Here's how the part is built. I have some questions about the finished solid (model axes, mm). Face numbers are marked on the shaded views. A direction names the side the tool comes from. Coordinates: 2 decimals unless noted, no trailing zeros. Write each loop counter-clockwise with the first axis right and the second up, starting at its lowest first coordinate (ties: lowest second). Pieces come first, ordered by that corner, then holes. Notation, with made-up numbers: (44.5, 19) - (66.5, 19) arc R18 ccw to (66.5, 29) - close; hole circle Ø6 at (30, 5). An arc over 180 degrees is marked (long way). Answer in a Markdown table with one row per item. Add a question column.
Item 1: Imagine slicing it at D-D (z = 20). Please give me the cut outline in (x, y), plus the area to 3 significant figures.
Item 2: Imagine slicing it at B-B (y = 0). Please give me the cut outline in (x, z) (3 decimals), plus the area to 3 significant figures.
Item 3: Imagine slicing it at C-C (z = 10). Please give me the cut outline in (x, y) (3 decimals), plus the area to 3 significant figures.
Item 4: If I drill on probe 1 along X at (y, z) = (0, 10.5) (3 decimals); probe 2 along Y at (x, z) = (2, 16.5); probe 3 along Y at (x, z) = (-2, 22), over which ranges is the centre line in solid material (lowest first)? Write a range as from..to.
Item 5: Imagine slicing it at A-A (x = 0). Please give me the cut outline in (y, z) (3 decimals), plus the area to 3 significant figures.
Item 6: Which directions (+Z, -Z, +X, -X, +Y, -Y) give clear straight access to the entire face, cutting with the end or side of a thin tool? Please do the marked faces 1 and 2.
Item 7: We'd pull the mould along X, two halves only. Please class the marked faces 3, 4, 5 and 6: +X half, -X half, draft (parallel to the pull), parting line (faces both ways), or undercut.
Item 8: I'm going to push flat-ended pins straight in: pin 1 (2 mm diameter, centred on y = -17, z = 27.5, fed in from +X); pin 2 (18.5 mm diameter, centred on y = 17.5, z = 15.5, fed in from -X); pin 3 (1.5 mm diameter, centred on x = -4, y = 19.5, fed in from -Z); pin 4 (1.5 mm diameter, centred on x = 0, y = 21.5, fed in from -Z). Where does each tip first touch, or does it pass through?
from build123d import *

# Parameters (mm, degrees)
PAD_DEPTH = 2.8


with BuildPart() as pad:
    # Sketch001 → Pad (new body, symmetric)
    with BuildSketch(Plane.YZ):
        with BuildLine():
            Line((6.5, 0), (6.5, 14))
            Line((6.5, 14), (10.5, 14))
            Line((10.5, 14), (17.86865, 27.377357))
            ThreePointArc((29.028201, 19.12997), (28.160419, 29.629469), (17.86865, 27.377357))
            Line((10.5, 0), (29.028201, 19.12997))
            Line((6.5, 0), (10.5, 0))
        make_face()
        with BuildLine():
            Line((-29.028193, 19.12994), (-10.49996, 0))
            Line((-10.49996, 0), (-6.49996, 0))
            Line((-6.49996, 0), (-6.49996, 14))
            Line((-6.49996, 14), (-10.49996, 14))
            Line((-10.49996, 14), (-17.86865, 27.377335))
            ThreePointArc((-17.86865, 27.377335), (-28.160423, 29.629443), (-29.028193, 19.12994))
        make_face()
    extrude(amount=PAD_DEPTH, both=True)


with BuildPart() as obj1:
    # Sketch → Revolution (revolve)
    with BuildSketch(Plane.YZ):
        Polygon((6, 0), (5.055, 0.545596), (5.055, 13.454404), (6, 14), (8.5, 14), (10, 0), align=None)
    revolve(axis=Axis((0, 0, 0), (0, 0, 1)))

    # Fusion: union Pad
    add(pad.part)


solid = obj1.part
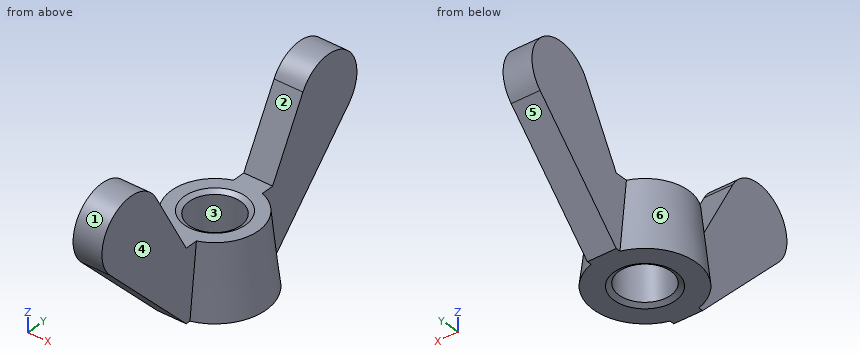
Here are the results:
| question | item | result |
|---|---|---|
| 1 | outline | (-2.8, -29.74) - (2.8, -29.74) - (2.8, -13.8) - (-2.8, -13.8) - close; (-2.8, 13.8) - (2.8, 13.8) - (2.8, 29.74) - (-2.8, 29.74) - close |
| 1 | area | 179 mm2 |
| 2 | outline | (-10, 0) - (-6, 0) - (-5.055, 0.546) - (-5.055, 13.454) - (-6, 14) - (-8.5, 14) - close; (5.055, 0.546) - (6, 0) - (10, 0) - (8.5, 14) - (6, 14) - (5.055, 13.454) - close |
| 2 | area | 116 mm2 |
| 3 | outline | (-2.8, -20.185) - (2.8, -20.185) - (2.8, -8.478) arc R8.929 ccw to (2.8, 8.478) - (2.8, 20.185) - (-2.8, 20.185) - (-2.8, 8.478) arc R8.929 ccw to (-2.8, -8.478) - close; hole circle Ø10.11 at (0, 0) |
| 3 | area | 298 mm2 |
| 4 | probe 1 | x = -8.875..-5.055, 5.055..8.875 |
| 4 | probe 2 | y = -26.48..-11.88, 11.88..26.48 |
| 4 | probe 3 | y = -30.71..-14.91, 14.91..30.71 |
| 5 | outline | (-29.028, 19.13) - (-10.5, 0) - (-6, 0) - (-5.055, 0.546) - (-5.055, 13.454) - (-6, 14) - (-10.5, 14) - (-17.869, 27.377) arc R7 ccw (long way) to start; (5.055, 0.546) - (6, 0) - (10.5, 0) - (29.028, 19.13) arc R7 ccw (long way) to (17.869, 27.377) - (10.5, 14) - (6, 14) - (5.055, 13.454) - close |
| 5 | area | 801 mm2 |
| 6 | face 1 | +X, -X |
| 6 | face 2 | +Z, +X, -X |
| 7 | face 3 | undercut |
| 7 | face 4 | +X half |
| 7 | face 5 | draft |
| 7 | face 6 | -X half |
| 8 | pin 1 | stops at x = 2.8 |
| 8 | pin 2 | stops at x = -2.8 |
| 8 | pin 3 | passes through |
| 8 | pin 4 | stops at z = 10.58 |
